```python
from build123d import *

# Parameters (mm, degrees)
F1_DEPTH  = 11
F2_R      = 28.523991
F3_R      = 5
F5_R      = 0.75
F5_R_2    = 4
F6_DEPTH  = 11.001
F7_R      = 4
F8_DEPTH  = 11.001
F10_DEPTH = 11.001


with BuildPart() as f1:
    # F0 (on Top) → F1 (new body)
    with BuildSketch(Plane.XY):
        with BuildLine():
            ThreePointArc((-59.119348, -199.42142), (-183.034682, -98.804378), (-199.158229, 60))
            Line((-199.158229, 60), (-222.036033, 60))
            ThreePointArc((-222.036033, 60), (0, -230), (222.036033, 60))
            Line((222.036033, 60), (199.158229, 60))
            ThreePointArc((199.158229, 60), (183.034682, -98.804378), (59.119348, -199.42142))
            Line((59.119348, -199.42142), (25, -188))
            Line((25, -188), (0, -188))
            Line((0, -188), (-25, -188))
            Line((-25, -188), (-59.119348, -199.42142))
        make_face()
    extrude(amount=F1_DEPTH)

    # F2
    f2_edges = [f1.edges().sort_by_distance(p)[0] for p in [
        (25, -188, 5.5),
        (-25, -188, 5.5),
    ]]
    fillet(f2_edges, radius=F2_R)

    # F3
    f3_edges = [f1.edges().sort_by_distance(p)[0] for p in [
        (59.119348, -199.42142, 5.5),
        (-59.119348, -199.42142, 5.5),
    ]]
    fillet(f3_edges, radius=F3_R)

    # F5 (on face) → F6 (cut, through all)
    with BuildSketch(Plane.XY.offset(11)):
        with Locations((0, -219)):
            Circle(F5_R)
        with Locations((48.732085, -213.509213)):
            Circle(F5_R)
        with Locations((95.020539, -197.312182)):
            Circle(F5_R)
        with Locations((136.544267, -171.221095)):
            Circle(F5_R)
        with Locations((171.221095, -136.544267)):
            Circle(F5_R)
        with Locations((197.312182, -95.020539)):
            Circle(F5_R)
        with Locations((213.509213, -48.732085)):
            Circle(F5_R)
        with Locations((219, 0)):
            Circle(F5_R)
        with Locations((213.509213, 48.732085)):
            Circle(F5_R)
        with Locations((197.312182, 95.020539)):
            Circle(F5_R)
        with Locations((171.221095, 136.544267)):
            Circle(F5_R)
        with Locations((136.544267, 171.221095)):
            Circle(F5_R)
        with Locations((95.020539, 197.312182)):
            Circle(F5_R)
        with Locations((48.732085, 213.509213)):
            Circle(F5_R)
        with Locations((0, 219)):
            Circle(F5_R)
        with Locations((-48.732085, 213.509213)):
            Circle(F5_R)
        with Locations((-95.020539, 197.312182)):
            Circle(F5_R)
        with Locations((-136.544267, 171.221095)):
            Circle(F5_R)
        with Locations((-171.221095, 136.544267)):
            Circle(F5_R)
        with Locations((-197.312182, 95.020539)):
            Circle(F5_R)
        with Locations((-213.509213, 48.732085)):
            Circle(F5_R)
        with Locations((-219, 0)):
            Circle(F5_R)
        with Locations((-213.509213, -48.732085)):
            Circle(F5_R)
        with Locations((-197.312182, -95.020539)):
            Circle(F5_R)
        with Locations((-171.221095, -136.544267)):
            Circle(F5_R)
        with Locations((-136.544267, -171.221095)):
            Circle(F5_R)
        with Locations((-95.020539, -197.312182)):
            Circle(F5_R)
        with Locations((-48.732085, -213.509213)):
            Circle(F5_R)
        with Locations((-5, -197)):
            Circle(F5_R)
        with Locations((5, -197)):
            Circle(F5_R)
        with Locations((0, -208)):
            Circle(F5_R)
        with Locations((-5, -217)):
            Circle(F5_R)
        with Locations((-25, -207)):
            Circle(F5_R)
        with Locations((5, -217)):
            Circle(F5_R)
        with Locations((25, -207)):
            Circle(F5_R)
        with Locations((-73.684961, -206.23173)):
            Circle(F5_R_2)
    extrude(amount=-F6_DEPTH, mode=Mode.SUBTRACT)

    # F7 (on face) → F8 (cut, through all)
    with BuildSketch(Plane.XY.offset(11)):
        with Locations((-171.221095, -136.544267)):
            Circle(F7_R)
        with Locations((171.221095, -136.544267)):
            Circle(F7_R)
    extrude(amount=-F8_DEPTH, mode=Mode.SUBTRACT)

    # F9 (on face) → F10 (cut, through all)
    with BuildSketch(Plane.XY.offset(11)):
        Polygon((0, 85.640151), (0, -188), (0, -205), (-5, -202.917908), (-5, -213.082092), (0, -211), (0, -251.474887), (263.787508, -251.474887), (263.787508, 85.640151), align=None)
    extrude(amount=-F10_DEPTH, mode=Mode.SUBTRACT)


solid = f1.part
```
Part model, mm, in its own coordinate system. A direction names the side the tool comes from. Coordinates: 2 decimals unless noted, no trailing zeros. Write each loop counter-clockwise with the first axis right and the second up, starting at its lowest first coordinate (ties: lowest second). Pieces come first, ordered by that corner, then holes.
Item 1: Which spindle directions (+Z, -Z, +X, -X, +Y, -Y) get a long thin tool onto all of the face, cutting with end or side? Do faces 4 (the face through (-43.31, -194.13, 5.42)), 5 (the face through (0, -215, 6)), 6 (the face through (-5, -208, 6)). Say none if no direction does.
Item 2: Mould opens along Y. For faces 1 (the face through (-71.84, -209.78, 5.58)), 2 (the face through (-158, -138, 11)), 3 (the face through (-10, -188, 5)) say: released by +Y, released by -Y, zero draft, split by the parting line, or undercut.
Item 3: Slice it at B-B (x = -150). Write the cut outline in (y, z), and give its area (3 significant figures).
Item 4: Slice it at C-C (y = -79.5). Write the cut outline in (x, z).
Item 5: Probe line 1 (Y direction, x = -71, z = 2.5); line 2 (X direction, y = -207, z = 5.5); line 3 (X direction, y = -126, z = 9.25). List the from-to ranges inside material, lowest first.
Item 6: Slice it at A-A (z = 3.25). Count the separate pieces of the cut face and the enclosed holes in it, and give its area (3 significant figures).
Item 7: Pin check, flat tips, straight feed: pin 1 (6 mm diameter, centred on x = -170.5, z = 6, fed in from -Y); pin 2 (3 mm diameter, centred on x = -170, z = 6, fed in from +Y); pin 3 (4 mm diameter, centred on x = -153, z = 5.5, fed in from -Y). Stop position of each tip, or through.
Results found:
1. face 4: +Z, -Z, +Y
1. face 5: +Z, -Z, +X, +Y, -Y
1. face 6: +Z, -Z
2. face 1: undercut
2. face 2: zero draft
2. face 3: released by +Y
3. outline: (-174.36, 0) - (-144.1, 0) - (-144.1, 11) - (-174.36, 11) - close
3. area: 333 mm2
4. outline: (-215.82, 0) - (-192.21, 0) - (-192.21, 11) - (-215.82, 11) - close
5. line 1: y = -218.77 to -209.2, -203.27 to -195.51
5. line 2: x = -100.25 to -77.61, -69.76 to -25.75, -24.25 to -5
5. line 3: x = -192.42 to -165.49
6. separate pieces: 1
6. enclosed holes: 12
6. area: 9,560 mm2
7. pin 1: stops at y = -157.62
7. pin 2: stops at y = -117.69
7. pin 3: stops at y = -173.49
